Autodesk Inventor part; units mm, degrees
ref_plane "YZ Plane" through (0, 0, 0) normal (1, 0, 0) x (0, 1, 0)
ref_plane "XZ Plane" through (0, 0, 0) normal (0, 1, 0) x (-1, 0, 0)
ref_plane "XY Plane" through (0, 0, 0) normal (0, 0, 1) x (1, 0, 0)
sketch "Sketch1" plane through (0, 0, 0) normal (0, 0, 1) x (1, 0, 0)
  line L0 (57, -12.5) -> (-57, -12.5)
  line L1 (-57, -12.5) -> (-57, 12.5)
  line L2 (-57, 12.5) -> (57, 12.5)
  line L3 (57, 12.5) -> (57, -12.5)
  line L4 (57, -12.5) -> (-57, 12.5) construction
  line L5 (-57, -12.5) -> (57, 12.5) construction
  point P0 (0, 0)
  dimension "d0" = 57
  dimension "d1" = 25
extrude "Extrusion1" add sketch "Sketch1" along normal blind 3
sketch "Sketch2" plane through (0, 0, 0) normal (0, 0, -1) x (-1, 0, 0)
  line L0 (57, 12.5) -> (57, -12.5)
  line L1 (57, 5) -> (60, 5)
  line L2 (60, 5) -> (60, -5)
  line L3 (60, -5) -> (57, -5)
  line L4 (57, -5) -> (57, 5)
  point P0 (0, 0)
  point P1 (60, 0)
  dimension "d4" = 3
  dimension "d5" = 10
extrude "Extrusion2" add sketch "Sketch2" against normal blind 3
sketch "Sketch3" plane through (0, 0, 0) normal (0, 0, -1) x (-1, 0, 0)
  line L0 (-57, -12.5) -> (57, -12.5)
  line L1 (50, -12.5) -> (30, -12.5)
  line L2 (30, -12.5) -> (30, -15.5)
  line L3 (30, -15.5) -> (50, -15.5)
  line L4 (50, -15.5) -> (50, -12.5)
  line L5 (-10, -12.5) -> (10, -12.5)
  line L6 (10, -12.5) -> (10, -15.5)
  line L7 (10, -15.5) -> (-10, -15.5)
  line L8 (-10, -15.5) -> (-10, -12.5)
  point P0 (0, 0)
  point P1 (0, -15.5)
  dimension "d8" = 20
  dimension "d9" = 3
  dimension "d10" = 30
  dimension "d11" = 20
  dimension "d12" = 3
  dimension "d13" = 20
extrude "Extrusion3" add sketch "Sketch3" against normal blind 3
properties part number "motor reinforcment"
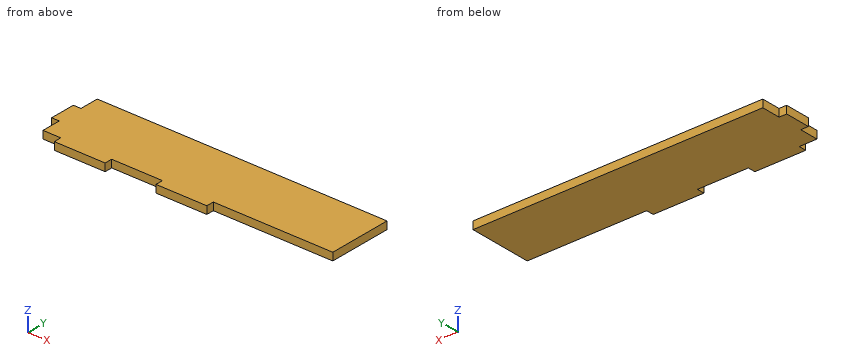
Build history of the part. All positions in model axes, mm. Give positions to 0.01 mm unless a question says otherwise; leave off trailing zeros. Order: outer loops, then holes, each group sorted by start corner. A loop starts at its lowest first (then second) coordinate and runs counter-clockwise, first axis right, second up. Notation, with made-up numbers: M 67,62 L 109,62 A30 cw 109,97 Z; hole C 30.25,-7.5 d2. An arc over 180 degrees is marked long. Write item = value, one per line. Start each with the question number.
(1) Slice it at A-A on y = -13.5. Write the cut outline in (x, z), plus the area to 3 significant figures.
(2) Pin check, flat tips, straight feed: pin 1 Ø1.5 at (y, z) = (-13.5, 1) entering from +X; pin 2 Ø0.9 at (x, z) = (-59, 2) entering from +Y; pin 3 Ø0.9 at (x, z) = (26.5, 1) entering from -Y; pin 4 Ø5 at (x, y) = (6, -11) entering from -Z. Stop position of each tip, or through.
(3) Slice it at B-B on z = 2.5. Write the cut outline in (x, y).
(4) Probe L1, parallel to X at y = -9.5, z = 0.55; L2, parallel to Y at x = 32.5, z = 1.65; L3, parallel to X at y = -13, z = 1.05. List the from-to ranges inside material, lowest first. Write a range as [from, to].
(5) Slice it at C-C on x = 16.5. Write the cut outline in (y, z), plus the area to 3 significant figures.
Responses:
q1.outline = M -50,0 L -30,0 L -30,3 L -50,3 Z; M -10,0 L 10,0 L 10,3 L -10,3 Z
q1.area = 120 mm2
q2.pin_1 = 10
q2.pin_2 = 5
q2.pin_3 = -12.5
q2.pin_4 = 0
q3.outline = M -60,-5 L -57,-5 L -57,-12.5 L -50,-12.5 L -50,-15.5 L -30,-15.5 L -30,-12.5 L -10,-12.5 L -10,-15.5 L 10,-15.5 L 10,-12.5 L 57,-12.5 L 57,12.5 L -57,12.5 L -57,5 L -60,5 Z
q4.L1 = [-57, 57]
q4.L2 = [-12.5, 12.5]
q4.L3 = [-50, -30], [-10, 10]
q5.outline = M -12.5,0 L 12.5,0 L 12.5,3 L -12.5,3 Z
q5.area = 75.0 mm2
